Input: part model. Units: mm. Frame: model coordinates. Face numbers are marked on the shaded views. A direction names the side the tool comes from. Round coordinates to 2 decimals unless told otherwise and drop trailing zeros. Order: outer loops, then holes, each group sorted by start corner. A loop starts at its lowest first (then second) coordinate and runs counter-clockwise, first axis right, second up.
Item 1: First-contact query: pin 1 (2.5 mm diameter, centred on x = 0.5, z = 0.5, fed in from -Y); pin 2 (6 mm diameter, centred on x = 3.5, y = 10, fed in from +Z); pin 3 (2 mm diameter, centred on y = 3.5, z = -1, fed in from +X); pin 4 (6 mm diameter, centred on x = -3.5, y = 20, fed in from -Z). Flat tips, straight axial feed; report the tip coordinate or a pass-through.
Item 2: Cut plane B-B on y = 17. Output: boundary loops of the cut face in (x, z).
Item 3: Line query: L1, parallel to X at y = 8, z = 0; L2, parallel to X at y = 20.5, z = 0; L3, parallel to Y at x = 4, z = -4.25. Output: solid intervals per line, ascending.
Item 4: Cut plane A-A on y = 2.5. Output: boundary loops of the cut face in (x, z).
Item 5: Reachability of the marked faces 4 and 5 from +Z, -Z, +X, -X, +Y, -Y: full face, straight path, thin tool, end or side. Return the list, or none.
Item 6: Mould query, pull axis X, two halves, no side actions, for the marked faces 1, 2 and 3. Classes: released by +X, released by -X, zero draft, split by the parting line, or undercut.
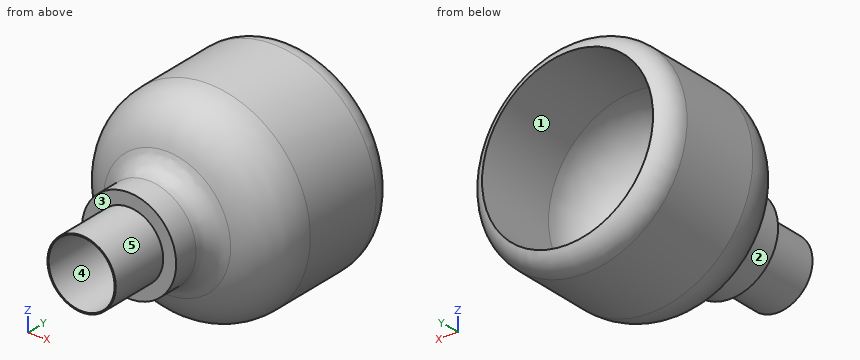
```python
from build123d import *

# Parameters (mm, degrees)
FILLET2_R           = 2
FILLET5_R           = 2
SKETCH4_R           = 2.9
SKETCH4_R_2         = 2.8
BOSS_EXTRUDE1_DEPTH = 5


with BuildPart() as part:
    # Sketch1 → Revolve1 (revolve)
    with BuildSketch(Plane.XY, mode=Mode.PRIVATE) as revolve1_sk:
        with BuildLine():
            Line((2.8, 5.768459657), (2.8, 11.536919315))
            ThreePointArc((2.8, 11.536919315), (5.949994158, 12.841689616), (7.254764459, 15.991683774))
            Line((7.254764459, 15.991683774), (7.254764459, 23.002625948))
            Line((7.254764459, 23.002625948), (8.614040085, 23.002625948))
            Line((8.614040085, 23.002625948), (8.614040085, 14.175242604))
            ThreePointArc((8.614040085, 14.175242604), (7.262619033, 10.912623572), (4, 9.56120252))
            Line((4, 9.56120252), (4, 5.768459657))
            Line((4, 5.768459657), (2.8, 5.768459657))
        make_face()
    revolve(revolve1_sk.sketch.rotate(Axis((0, 81.429038173, 0), (0, -1, 0)), 90), axis=Axis((0, 81.429038173, 0), (0, -1, 0)))

    # Fillet2
    # the kernel refuses this fillet: 2 mm, written as the material it takes off along each edge
    with BuildSketch(Plane(origin=(0, 23.002625948, 0), x_dir=(0, 0, 1), z_dir=(1, 0, 0))) as fillet2_piece_1:
        with BuildLine():
            CenterArc((6.614040085, 1.894590266), FILLET2_R, 288.684829844, 71.315170156)
            Line((8.614040085, 1.894590266), (8.654040085, 1.894590266))
            Line((8.654040085, 1.894590266), (8.654040085, 0))
            Line((8.654040085, 0), (8.614040085, -0.04))
            ThreePointArc((8.614040085, -0.04), (7.934402272, -0.04), (7.267578947, -0.037891805))
            Line((7.267578947, -0.037891805), (7.254764459, 0))
        make_face()
    revolve(axis=Axis((0, 23.002625948, 0), (0, -1, 0)), mode=Mode.SUBTRACT)

    # Fillet5
    fillet5_edges = [part.edges().sort_by_distance(p)[0] for p in [
        (0, 9.56120252, -4),
    ]]
    fillet(fillet5_edges, radius=FILLET5_R)

    # Sketch4 → Boss-Extrude1 (add)
    with BuildSketch(Plane.XZ.offset(-5.768459657)):
        with Locations(Location((0, 0, 0), (0, 0, 90))):
            Circle(SKETCH4_R)
        with Locations(Location((0, 0, 0), (0, 0, 90))):
            Circle(SKETCH4_R_2, mode=Mode.SUBTRACT)
    extrude(amount=BOSS_EXTRUDE1_DEPTH)


solid = part.part
```
From the geometry:
1. pin 1: passes through
1. pin 2: stops at z = 8.09
1. pin 3: stops at x = 2.9
1. pin 4: stops at z = -8.6
2. outline: circle Ø17.23 at (0, 0); hole circle Ø14.51 at (0, 0)
3. L1: x = -4 to -2.8, 2.8 to 4
3. L2: x = -8.61 to -7.25, 7.25 to 8.61
3. L3: y = 9.94 to 12.73
4. outline: circle Ø5.8 at (0, 0); hole circle Ø5.6 at (0, 0)
5. face 4: +Y, -Y
5. face 5: -Y
6. face 1: undercut
6. face 2: split by the parting line
6. face 3: zero draft
